Work out the finished part from the listing and answer in its coordinate system (mm). A direction names the side the tool comes from. Round coordinates to 2 decimals unless told otherwise and drop trailing zeros. Write each loop counter-clockwise with the first axis right and the second up, starting at its lowest first coordinate (ties: lowest second). Pieces come first, ordered by that corner, then holes. Notation, with made-up numbers: M -32,9.25 L -5,9.25 A30 cw -5,38.25 Z; hole C 19,-38 d10. An arc over 180 degrees is marked long. Answer in a Markdown table with one row per item.
```python
from build123d import *

# Parameters (mm, degrees)
SKETCH1_R           = 4
BOSS_EXTRUDE4_DEPTH = 5
SKETCH4_W           = 40
SKETCH4_H           = 5
BOSS_EXTRUDE5_DEPTH = 30
BOSS_EXTRUDE6_START = 5
SKETCH5_W           = 40
SKETCH5_H           = 5
SKETCH5_R           = 4
BOSS_EXTRUDE6_DEPTH = 5
SKETCH7_R           = 3
CUT_EXTRUDE1_DEPTH  = 15


with BuildPart() as part:
    # Sketch1 → Boss-Extrude4 (new body)
    with BuildSketch(Plane.XY):
        with BuildLine():
            Line((-20, -35), (20, -35))
            Line((20, -35), (20, 5))
            ThreePointArc((20, 5), (17.071067812, 12.071067812), (10, 15))
            Line((10, 15), (-10, 15))
            ThreePointArc((-10, 15), (-17.071067812, 12.071067812), (-20, 5))
            Line((-20, 5), (-20, -35))
        make_face()
        Circle(SKETCH1_R, mode=Mode.SUBTRACT)
    extrude(amount=BOSS_EXTRUDE4_DEPTH)

    # Sketch4 → Boss-Extrude5 (add)
    with BuildSketch(Plane(origin=(0, 0, 0), x_dir=(-1, 0, 0), z_dir=(0, 0, -1))):
        with Locations((0, -32.5)):
            Rectangle(SKETCH4_W, SKETCH4_H)
    extrude(amount=BOSS_EXTRUDE5_DEPTH)

    # Sketch5 → Boss-Extrude6 (add)
    # profile 1 of 2: a face of its own
    with BuildSketch(Plane(origin=(0, 0, -30), x_dir=(-1, 0, 0), z_dir=(0, 0, -1)).offset(BOSS_EXTRUDE6_START)):
        with Locations((0, -32.5)):
            Rectangle(SKETCH5_W, SKETCH5_H)
    # profile 2 of 2: a face of its own
    with BuildSketch(Plane(origin=(0, 0, -30), x_dir=(-1, 0, 0), z_dir=(0, 0, -1)).offset(BOSS_EXTRUDE6_START)):
        with BuildLine():
            Line((-20, 0), (-20, -30))
            Line((-20, -30), (20, -30))
            Line((20, -30), (20, 0))
            Line((20, 0), (20, 5))
            ThreePointArc((20, 5), (17.071067812, 12.071067812), (10, 15))
            Line((10, 15), (-10, 15))
            ThreePointArc((-10, 15), (-17.071067812, 12.071067812), (-20, 5))
            Line((-20, 5), (-20, 0))
        make_face()
        with Locations(Location((0, 0, 0), (0, 0, 180))):
            Circle(SKETCH5_R, mode=Mode.SUBTRACT)
    extrude(amount=-BOSS_EXTRUDE6_DEPTH)

    # Sketch7 → Cut-Extrude1 (cut)
    with BuildSketch(Plane(origin=(0, -30, 0), x_dir=(1, 0, 0), z_dir=(0, 1, 0))):
        with Locations(Location((-7, 15, 0), (0, 0, 270))):
            Circle(SKETCH7_R)
        with Locations(Location((7, 15, 0), (0, 0, 270))):
            Circle(SKETCH7_R)
    extrude(amount=-CUT_EXTRUDE1_DEPTH, mode=Mode.SUBTRACT)


solid = part.part
```
1. The part is cut by section C-C (z = -32). Determine the outline of the cut face in (x, y), plus the area to 3 significant figures.
Calculated:
| item | result |
|---|---|
| outline | M -20,-35 L 20,-35 L 20,5 A10 ccw 10,15 L -10,15 A10 ccw -20,5 Z; hole C 0,0 d8 |
| area | 1,910 mm² |
2. The part is cut by section B-B (x = 0). Determine the outline of the cut face in (y, z).
Calculated:
| item | result |
|---|---|
| outline | M -35,-35 L -4,-35 L -4,-30 L -30,-30 L -30,0 L -4,0 L -4,5 L -35,5 Z; M 4,-35 L 15,-35 L 15,-30 L 4,-30 Z; M 4,0 L 15,0 L 15,5 L 4,5 Z |
3. The part is cut by section A-A (x = -7). Determine the outline of the cut face in (y, z).
Calculated:
| item | result |
|---|---|
| outline | M -35,-35 L 15,-35 L 15,-30 L -30,-30 L -30,-18 L -35,-18 Z; M -35,-12 L -30,-12 L -30,0 L 15,0 L 15,5 L -35,5 Z |
4. Given pin 1 (9 mm diameter, centred on x = 0, y = 0, fed in from -Z); pin 2 (1.5 mm diameter, centred on x = -1.5, z = -27, fed in from +Y), each flat-ended and moving along its own axis, determine where each tip first touches the part or whether it passes through.
Calculated:
| item | result |
|---|---|
| pin 1 | stops at z = -35 |
| pin 2 | stops at y = -30 |
5. A tool of negligible diameter and unlimited length cuts with its end or side. For faces 1 (the flat face through (0, -30, -15)), 2 (the flat face through (0, -35, -15)), from which of +Z, -Z, +X, -X, +Y, -Y can it reach the whole face along a straight path? Write none if from no direction.
Calculated:
| item | result |
|---|---|
| face 1 | +X, -X, +Y |
| face 2 | +Z, -Z, +X, -X, -Y |
6. Consider line 1 along X through (y, z) = (-31, -15); line 2 along Y through (x, z) = (0, 2.7); line 3 along Z through (x, y) = (9.5, 13). Determine where each line is inside the solid, lowest interval first. Write a range as from..to.
Calculated:
| item | result |
|---|---|
| line 1 | x = -20..-10, -4..4, 10..20 |
| line 2 | y = -35..-4, 4..15 |
| line 3 | z = -35..-30, 0..5 |
7. The part is cut by section D-D (z = -15). Determine the outline of the cut face in (x, y), plus the area to 3 significant figures.
Calculated:
| item | result |
|---|---|
| outline | M -20,-35 L -10,-35 L -10,-30 L -20,-30 Z; M -4,-35 L 4,-35 L 4,-30 L -4,-30 Z; M 10,-35 L 20,-35 L 20,-30 L 10,-30 Z |
| area | 140 mm² |
8. Determine the mould class of faces 3 (the flat face through (0, -7, -30)), 4 (the cylindrical face through (5.2, -32.5, -17.4)), 5 (the flat face through (0, -10, -35)), 6 (the cylindrical face through (16.99, 12.15, -32.53)) for opening direction Z: released by +Z, released by -Z, zero draft, split by the parting line, or undercut.
Calculated:
| item | result |
|---|---|
| face 3 | undercut |
| face 4 | undercut |
| face 5 | released by -Z |
| face 6 | zero draft |
